```python
from build123d import *

# Parameters (mm, degrees)
M2_TAPPED_HOLE1_AT_2_COUNT = 2
M2_TAPPED_HOLE1_AT_2_PITCH = 11.313708499
M2_TAPPED_HOLE1_AT_3_COUNT = 2
M2_TAPPED_HOLE1_AT_3_PITCH = 16
M2_TAPPED_HOLE1_AT_4_COUNT = 2
M2_TAPPED_HOLE1_AT_4_PITCH = 11.313708499
M2_TAPPED_HOLE1_AT_5_COUNT = 2
M2_TAPPED_HOLE1_AT_5_PITCH = 8
RADYUS1_R                  = 0.5
IZIM1_R                    = 1.025
KES_EKSTR_ZYON1_DEPTH      = 10


with BuildPart() as part:
    # Sketch1 → Revolve1 (revolve)
    with BuildSketch(Plane(origin=(0, 0, 0), x_dir=(0, 0, -1), z_dir=(1, 0, 0))):
        Polygon((2.5, 1.25), (1, 1.25), (1, 2.75), (0, 2.75), (0, 11), (3, 11), (3, 2.75), (2.5, 2.75), align=None)
    revolve(axis=Axis((0, 0, 0), (0, 0, 1)))

    # Sketch4 → M2 Tapped Hole1 (revolve, cut)
    with BuildSketch(Plane(origin=(0, 8, 0), x_dir=(0, -1, 0), z_dir=(1, 0, 0))):
        Polygon((0, 0), (0, 3), (1.025, 3), (0.8, 2.870096189), (0.8, 0.129903811), (1.025, 0), align=None)
    m2_tapped_hole1 = revolve(axis=Axis((0, 8, 6.35), (0, 0, -1)), mode=Mode.SUBTRACT)

    # M2 Tapped Hole1 at 2: M2 Tapped Hole1 ×2
    with Locations(*[Vector(0.707106781, -0.707106781, 0) * (i * M2_TAPPED_HOLE1_AT_2_PITCH) for i in range(1, M2_TAPPED_HOLE1_AT_2_COUNT)]):
        add(m2_tapped_hole1, mode=Mode.SUBTRACT)

    # M2 Tapped Hole1 at 3: M2 Tapped Hole1 ×2
    with Locations(*[(0, -i * M2_TAPPED_HOLE1_AT_3_PITCH, 0) for i in range(1, M2_TAPPED_HOLE1_AT_3_COUNT)]):
        add(m2_tapped_hole1, mode=Mode.SUBTRACT)

    # M2 Tapped Hole1 at 4: M2 Tapped Hole1 ×2
    with Locations(*[Vector(-0.707106781, -0.707106781, 0) * (i * M2_TAPPED_HOLE1_AT_4_PITCH) for i in range(1, M2_TAPPED_HOLE1_AT_4_COUNT)]):
        add(m2_tapped_hole1, mode=Mode.SUBTRACT)

    # M2 Tapped Hole1 at 5: M2 Tapped Hole1 ×2
    with Locations(*[(0, -i * M2_TAPPED_HOLE1_AT_5_PITCH, 0) for i in range(1, M2_TAPPED_HOLE1_AT_5_COUNT)]):
        add(m2_tapped_hole1, mode=Mode.SUBTRACT)

    # Radyus1
    radyus1_edges = [part.edges().sort_by_distance(p)[0] for p in [
        (0, -11, -3),
        (0, -11, 0),
    ]]
    fillet(radyus1_edges, radius=RADYUS1_R)

    # Çizim1 → Kes-Ekstrüzyon1 (cut)
    with BuildSketch(Plane.XY):
        with Locations((0, 8)):
            Circle(IZIM1_R)
        with Locations((-8, 0)):
            Circle(IZIM1_R)
        with Locations((8, 0)):
            Circle(IZIM1_R)
        with Locations((0, -8)):
            Circle(IZIM1_R)
    extrude(amount=-KES_EKSTR_ZYON1_DEPTH, mode=Mode.SUBTRACT)


solid = part.part
```
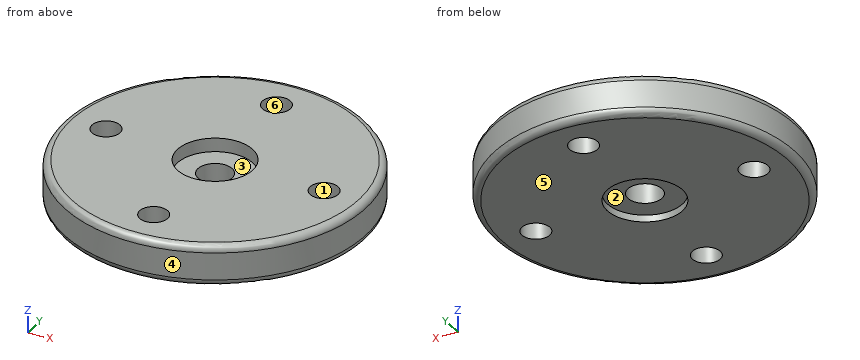
The model under review builds one solid part; all positions refer to its coordinate system, in mm. Face numbers are marked on the shaded views. A direction names the side the tool comes from. Give positions to 0.01 mm unless a question says otherwise; leave off trailing zeros. Write each loop counter-clockwise with the first axis right and the second up, starting at its lowest first coordinate (ties: lowest second). Pieces come first, ordered by that corner, then holes. Notation, with made-up numbers: (-7, 23.25) - (0, 23.25) arc R19 cw to (0, 49.25) - close; hole circle Ø5 at (60, 67.25). An arc over 180 degrees is marked (long way). Answer in a Markdown table with one row per item. Add a question column.
1. We need section B-B on z = -1.4. Write out the cut boundary in (x, y) (3 decimals).
2. Wall thickness on line 1 along Y through (x, z) = (0, -2.1) (3 decimals); line 2 along Y through (x, z) = (0.75, -0.5); line 3 along X through (y, z) = (-8.75, -2.3): over which ranges is each line inside the solid? List them lowest first. Write a range as [from, to].
3. We need section A-A on y = 0. Write out the cut boundary in (x, z) (3 decimals), then the cut area to 3 significant figures.
4. Insertion check: P1, Ø1, axis at x = -3.5, z = -0.5, coming from the -Y side; P2, Ø9, axis at x = 0, y = 0, coming from the -Z side; P3, Ø3, axis at x = 0, y = 0, coming from the -Z side; P4, Ø5, axis at x = 0, y = 0, coming from the +Z side. Each pin has a flat end and moves straight along its axis. Give the tip position at first contact, or say it passes through.
5. Tool access review of the marked faces 1, 2 and 3: name each direction out of +Z, -Z, +X, -X, +Y, -Y from which nothing blocks a thin tool from reaching the whole face with its end or side.
6. Draft analysis for pull direction Y (two halves, no side actions). For the marked faces 4, 5 and 6, state which applies: +Y half, -Y half, draft (parallel to the pull), parting line (faces both ways), or undercut.
Ans:
| question | item | result |
|---|---|---|
| 1 | outline | circle Ø22 at (0, 0); hole circle Ø2.05 at (-8, 0); hole circle Ø2.5 at (0, 0); hole circle Ø2.05 at (0, -8); hole circle Ø2.05 at (0, 8); hole circle Ø2.05 at (8, 0) |
| 2 | line 1 | y = [-11, -9.025], [-6.975, -1.25], [1.25, 6.975], [9.025, 11] |
| 2 | line 2 | y = [-10.97, -8.7], [-7.3, -2.65], [2.65, 7.3], [8.7, 10.97] |
| 2 | line 3 | x = [-6.67, -0.7], [0.7, 6.67] |
| 3 | outline | (-11, -2.5) arc R0.5 ccw to (-10.5, -3) - (-9.025, -3) - (-9.025, 0) - (-10.5, 0) arc R0.5 ccw to (-11, -0.5) - close; (-6.975, -3) - (-2.75, -3) - (-2.75, -2.5) - (-1.25, -2.5) - (-1.25, -1) - (-2.75, -1) - (-2.75, 0) - (-6.975, 0) - close; (1.25, -2.5) - (2.75, -2.5) - (2.75, -3) - (6.975, -3) - (6.975, 0) - (2.75, 0) - (2.75, -1) - (1.25, -1) - close; (9.025, -3) - (10.5, -3) arc R0.5 ccw to (11, -2.5) - (11, -0.5) arc R0.5 ccw to (10.5, 0) - (9.025, 0) - close |
| 3 | area | 41.5 mm^2 |
| 4 | P1 | stops at y = -10.58 |
| 4 | P2 | stops at z = -3 |
| 4 | P3 | stops at z = -2.5 |
| 4 | P4 | stops at z = -1 |
| 5 | face 1 | +Z, -Z |
| 5 | face 2 | -Z |
| 5 | face 3 | +Z |
| 6 | face 4 | parting line |
| 6 | face 5 | draft |
| 6 | face 6 | undercut |
